Can you work these out from the model? Positions are in its coordinate system, mm. Face numbers are marked on the shaded views. A direction names the side the tool comes from. Give positions to 0.01 mm unless a question says otherwise; leave off trailing zeros. Loops run counter-clockwise (first coordinate to the right, second up) from the corner with the lowest first, then second, coordinate; pieces in that order, holes last. Notation, with made-up numbers: (29, -20) - (84, -20) arc R33 ccw to (84, 16) - close; hole circle Ø7 at (76.25, 5). An arc over 180 degrees is marked (long way). Answer as a JSON object with one key per item and string values. Group by question number.
Item 1: Which directions (+Z, -Z, +X, -X, +Y, -Y) give clear straight access to the entire face, cutting with the end or side of a thin tool? Please do the marked faces 1, 2 and 3.
Item 2: Suppose I cut it at D-D on z = 83. Write out the boundary of the cut face in (x, y).
Item 3: Thinking about a two-plate mould opening in X: for the marked faces 4, 5 and 6, which applies, pulls with the +X half, pulls with the -X half, needs draft (parallel to the pull), parting line crosses it, or undercut?
Item 4: Please list where these lines run through material, in increasing order: L1, parallel to Z at x = -124, y = 75.5; L2, parallel to Y at x = -50, z = 27; L3, parallel to X at y = 6, z = 104.5.
Item 5: Suppose I cut it at A-A on x = -80. Write out the boundary of the cut face in (y, z), and give its area (3 significant figures).
Item 6: Suppose I cut it at C-C on x = -60. Write out the boundary of the cut face in (y, z), and give its area (4 significant figures).
Item 7: Will these pins go through, and if not, where does the flat tip stop? pin 1 (2 mm diameter, centred on y = 26.5, z = 50, fed in from -X); pin 2 (6 mm diameter, centred on x = -67.47, z = 27.53, fed in from +Y).
Item 8: Suppose I cut it at B-B on z = 97.53. Write out the boundary of the cut face in (x, y), and give its area (3 significant figures).
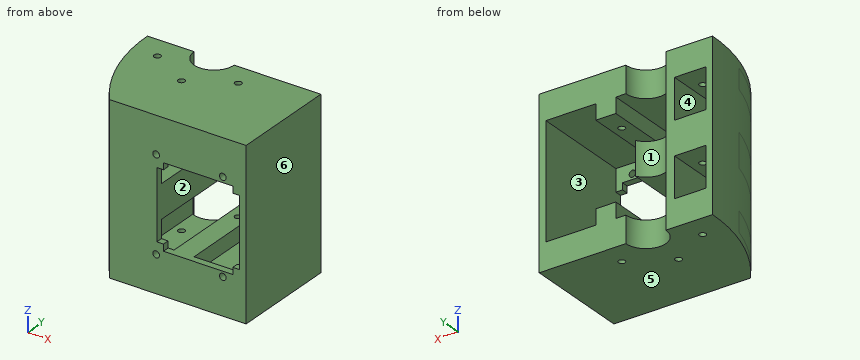
Autodesk Inventor part; units mm, degrees
ref_plane "YZ Plane" through (0, 0, 0) normal (1, 0, 0) x (0, 1, 0)
ref_plane "XZ Plane" through (0, 0, 0) normal (0, 1, 0) x (-1, 0, 0)
ref_plane "XY Plane" through (0, 0, 0) normal (0, 0, 1) x (1, 0, 0)
sketch "Sketch1" plane through (0, 0, 0) normal (0, 0, 1) x (1, 0, 0)
  circle A0 centre (0, 80) radius 130 construction
  line L0 (0, -50) -> (0, 0) construction
  line L1 (0, 0) -> (-102.4695, 0) construction
  arc A1 (-130, 80) -> (-102.4695, 0) centre (0, 80) ccw
  line L2 (-130, 80) -> (0, 80)
  line L3 (0, 80) -> (0, 0)
  line L4 (-102.4695, 0) -> (0, 0)
  dimension "d0" = 260
  dimension "d1" = 50
extrude "Extrusion1" add sketch "Sketch1" along normal blind 125
sketch "Sketch6" plane through (-130, 80, 0) normal (0, 1, 0) x (1, 0, 0)
  line L0 (0, 0) -> (0, -125)
  line L1 (0, 0) -> (130, 0)
  line L2 (130, 0) -> (130, -125)
  line L3 (130, -125) -> (0, -125)
  line L4 (0, -125) -> (0, 0)
  line L5 (5, -120) -> (125, -120)
  line L6 (125, -120) -> (125, -5)
  line L7 (125, -5) -> (5, -5)
  line L8 (5, -5) -> (5, -120)
  point P0 (130, 0)
  dimension "d25" = 5
extrude "Extrusion5" cut sketch "Sketch6" against normal blind 75 contours L8 L7 L6 L5
sketch "Sketch7" plane through (-102.4695, 0, 0) normal (0, -1, 0) x (1, 0, 0)
  circle A0 centre (35, 97.53) radius 2.5
  circle A1 centre (85, 97.53) radius 2.5
  line L0 (0, 125) -> (102.4695, 125)
  line L1 (0, 0) -> (0, 125)
  circle A2 centre (35, 27.53) radius 2.5
  circle A3 centre (85, 27.53) radius 2.5
  line L2 (102.4695, 0) -> (102.4695, 125)
  dimension "d28" = 5
  dimension "d29" = 5
  dimension "d30" = 27.47
  dimension "d31" = 50
  dimension "d33" = 5
  dimension "d34" = 5
  dimension "d35" = 70
  dimension "d82" = 35
extrude "Extrusion6" cut sketch "Sketch7" against normal through all
sketch "Sketch8" plane through (0, 0, 125) normal (0, 0, 1) x (1, 0, 0)
  line L0 (0, 80) -> (-130, 80)
  arc A0 (-130, 80) -> (-102.4695, 0) centre (0, 80) ccw
  arc A1 (-130, 80) -> (-102.4695, 0) centre (9.9581, 83.4269) ccw
  line L1 (-102.4695, 0) -> (-97.4695, 0)
  line L2 (-102.4695, 0) -> (0, 0)
  line L3 (-130, 80) -> (-125, 80)
  arc A2 (-125, 80) -> (-97.4695, 0) centre (14.9581, 83.4269) ccw
  dimension "d40" = 5
  dimension "d41" = 5
  dimension "d42" = 140
extrude "Extrusion7" add sketch "Sketch8" against normal blind 125
sketch "Sketch11" plane through (-130, 5, 0) normal (0, 1, 0) x (1, 0, 0)
  line L0 (125, -5) -> (125, -120)
  line L1 (125, -50) -> (5, -50)
  line L2 (5, -50) -> (5, -65)
  line L3 (5, -65) -> (125, -65)
  line L4 (125, -65) -> (125, -50)
  line L5 (125, -60) -> (5, -60)
  line L6 (5, -60) -> (5, -75)
  line L7 (5, -75) -> (125, -75)
  line L8 (125, -75) -> (125, -60)
  line L9 (32.7619, 0) -> (32.7619, -150)
  line L10 (125, -105) -> (5, -105)
  line L11 (5, -105) -> (5, -120)
  line L12 (5, -120) -> (125, -120)
  line L13 (125, -120) -> (125, -105)
  line L14 (125, -20) -> (5, -20)
  line L15 (5, -20) -> (5, -5)
  line L16 (5, -5) -> (125, -5)
  line L17 (125, -5) -> (125, -20)
  line L18 (5, -5) -> (125, -5)
  line L19 (5, -120) -> (5, -5)
  line L20 (125, -120) -> (5, -120)
  line L21 (125, -5) -> (125, -20)
  point P0 (130, 0)
  point P1 (65, -120)
  point P2 (65, -5)
  point P3 (5, -12.5)
  point P4 (5, -57.5)
  dimension "d54" = 15
  dimension "d55" = 15
  dimension "d56" = 15
  dimension "d57" = 15
  dimension "d58" = 30
  dimension "d59" = 30
  dimension "d66" = 5
extrude "Extrusion10" add sketch "Sketch11" along normal blind 75 contours L0 L14 L9 L16 | L9 L14 L15 L16 | L0 L5 L9 L1 | L0 L3 L9 L5 | L9 L5 L2 L1 | L0 L7 L9 L3 | L9 L3 L2 L5 | L9 L7 L6 L3 | L0 L12 L9 L10 | L9 L12 L11 L10
sketch "Sketch12" plane through (-130, 5, 0) normal (0, 1, 0) x (1, 0, 0)
  line L0 (27.5305, 0) -> (130, 0)
  line L1 (27.5305, -125) -> (130, -125)
  line L2 (72.5, 0) -> (87.5, 0)
  line L3 (87.5, 0) -> (87.5, -125)
  line L4 (87.5, -125) -> (72.5, -125)
  line L5 (72.5, -125) -> (72.5, 0)
  line L6 (28.5256, 0) -> (43.5256, 0)
  line L7 (43.5256, 0) -> (43.5256, -125)
  line L8 (43.5256, -125) -> (28.5256, -125)
  line L9 (28.5256, -125) -> (28.5256, 0)
  line L10 (130, 0) -> (130, -125)
  dimension "d62" = 15
  dimension "d63" = 15
  dimension "d92" = 42.5
extrude "Extrusion11" add sketch "Sketch12" along normal blind 75 contours L0 L7 L1 L9 | L0 L3 L1 L5
sketch "Sketch9" plane through (0, 0, 125) normal (0, 0, 1) x (1, 0, 0)
  circle A0 centre (-80, 80) radius 15
  point P0 (0, 0)
  point P1 (0, 80)
  dimension "d45" = 30
  dimension "d46" = 80
extrude "Extrusion8" cut sketch "Sketch9" against normal through all
sketch "Sketch13" plane through (0, 0, 0) normal (0, 0, -1) x (-1, 0, 0)
  arc A0 (102.4695, 0) -> (130, 80) centre (-9.9581, 83.4269) ccw
  line L0 (130, 80) -> (130, 80)
  arc A1 (102.4695, 0) -> (130, 80) centre (0, 80) ccw
  line L1 (130, 80) -> (130, 80)
  line L2 (95, 80) -> (130, 80)
  line L3 (130, 80) -> (130, 0)
  line L4 (130, 0) -> (102.4695, 0)
  point P0 (0, 0)
  dimension "d67" = 140
extrude "Extrusion12" cut sketch "Sketch13" against normal through all contours A1 L3 L4
sketch "Sketch14" plane through (0, 0, 125) normal (0, 0, 1) x (1, 0, 0)
  line L0 (-102.4695, 0) -> (0, 0) construction
  circle A0 centre (-110.3109, 97.5) radius 2.5
  circle A1 centre (-80, 80) radius 35 construction
  circle A2 centre (-110.3109, 62.5) radius 2.5
  circle A3 centre (-80, 45) radius 2.5
  circle A4 centre (-49.6891, 62.5) radius 2.5
  circle A5 centre (-49.6891, 97.5) radius 2.5
  circle A6 centre (-80, 115) radius 2.5
  arc A7 (-95, 80) -> (-65, 80) centre (-80, 80) ccw
  point P0 (0, 80)
  dimension "d74" = 70
  dimension "d72" = 5
  dimension "d77" = 360
extrude "Extrusion13" cut sketch "Sketch14" against normal through all
sketch "Sketch16" plane through (-102.4695, 0, 0) normal (0, -1, 0) x (1, 0, 0)
  line L0 (35.4695, 31.5) -> (35.4695, 93.5) construction
  line L1 (97.4695, 93.5) -> (35.4695, 93.5) construction
  line L2 (35.4695, 93.5) -> (35.4695, 31.5) construction
  line L3 (35.4695, 31.5) -> (97.4695, 31.5) construction
  line L4 (97.4695, 31.5) -> (97.4695, 93.5) construction
  line L5 (0, 125) -> (102.4695, 125)
  line L6 (0, 0) -> (102.4695, 0)
  line L7 (102.4695, 0) -> (102.4695, 125)
  line L8 (97.4695, 93.5) -> (92.4695, 93.5) construction
  line L9 (92.4695, 93.5) -> (92.4695, 88.5) construction
  line L10 (92.4695, 88.5) -> (97.4695, 88.5) construction
  line L11 (97.4695, 88.5) -> (97.4695, 93.5) construction
  line L12 (35.4695, 31.5) -> (40.4695, 31.5) construction
  line L13 (40.4695, 31.5) -> (40.4695, 36.5) construction
  line L14 (40.4695, 36.5) -> (35.4695, 36.5) construction
  line L15 (35.4695, 36.5) -> (35.4695, 31.5) construction
  line L16 (35.4695, 93.5) -> (40.4695, 93.5) construction
  line L17 (40.4695, 93.5) -> (40.4695, 88.5) construction
  line L18 (40.4695, 88.5) -> (35.4695, 88.5) construction
  line L19 (35.4695, 88.5) -> (35.4695, 93.5) construction
  line L20 (97.4695, 31.5) -> (92.4695, 31.5) construction
  line L21 (92.4695, 31.5) -> (92.4695, 36.5) construction
  line L22 (92.4695, 36.5) -> (97.4695, 36.5) construction
  line L23 (97.4695, 36.5) -> (97.4695, 31.5) construction
  line L24 (92.4695, 93.5) -> (40.4695, 93.5)
  line L25 (40.4695, 88.5) -> (40.4695, 93.5)
  line L26 (35.4695, 88.5) -> (40.4695, 88.5)
  line L27 (35.4695, 88.5) -> (35.4695, 36.5)
  line L28 (35.4695, 36.5) -> (40.4695, 36.5)
  line L29 (40.4695, 36.5) -> (40.4695, 31.5)
  line L30 (40.4695, 31.5) -> (92.4695, 31.5)
  line L31 (92.4695, 31.5) -> (92.4695, 36.5)
  line L32 (92.4695, 36.5) -> (97.4695, 36.5)
  line L33 (97.4695, 20) -> (97.4695, 50)
  line L34 (97.4695, 36.5) -> (97.4695, 88.5)
  line L35 (97.4695, 75) -> (97.4695, 105)
  line L36 (92.4695, 88.5) -> (97.4695, 88.5)
  line L37 (92.4695, 88.5) -> (92.4695, 93.5)
  point P0 (97.4695, 62.5)
  point P1 (102.4695, 62.5)
  point P2 (66.4695, 31.5)
  point P3 (51.2348, 0)
  dimension "d100" = 62
  dimension "d101" = 62
  dimension "d102" = 5
  dimension "d103" = 5
  dimension "d104" = 5
  dimension "d105" = 5
  dimension "d106" = 5
  dimension "d107" = 5
  dimension "d108" = 5
  dimension "d109" = 5
  dimension "d110" = 5
extrude "Extrusion15" cut sketch "Sketch16" against normal through all
equation "\"d101\" = d100"
properties part number "SJ005" material "ABS Plastic"
Worked out:
{
 "1": {"face 1": "+Z, -Z, +Y", "face 2": "+Y, -Y", "face 3": "+Y"},
 "2": {"outline": "(-130, 80) arc R130 ccw to (-102.47, 0) - (-67, 0) - (-67, 5) - (-86.47, 5) - (-86.47, 66.47) arc R15 cw to (-95, 80) - (-101.47, 80) - (-101.47, 5.69) arc R140 cw to (-125, 80) - close; (-5, 0) - (0, 0) - (0, 80) - (-5, 80) - close"},
 "3": {"face 4": "undercut", "face 5": "needs draft", "face 6": "pulls with the +X half"},
 "4": {"L1": "z = 0 to 20, 50 to 75, 105 to 125", "L2": "y = 0 to 60.02, 64.98 to 80", "L3": "x = -106.88 to -101.68, -101.47 to -86.47, -57.5 to -42.5, -5 to 0"},
 "5": {"outline": "(0, 0) - (42.5, 0) - (42.5, 20) - (5, 20) - (5, 50) - (42.5, 50) - (42.5, 75) - (5, 75) - (5, 105) - (42.5, 105) - (42.5, 125) - (0, 125) - close; (47.5, 0) - (65, 0) - (65, 20) - (47.5, 20) - close; (47.5, 50) - (65, 50) - (65, 75) - (47.5, 75) - close; (47.5, 105) - (65, 105) - (65, 125) - (47.5, 125) - close", "area": "4,200 mm2"},
 "6": {"outline": "(0, 0) - (80, 0) - (80, 20) - (5, 20) - (5, 31.5) - (0, 31.5) - close; (0, 93.5) - (5, 93.5) - (5, 105) - (80, 105) - (80, 125) - (0, 125) - close", "area": "3,315 mm2"},
 "7": {"pin 1": "stops at x = -118.93", "pin 2": "stops at y = 5"},
 "8": {"outline": "(-130, 80) arc R130 ccw to (-102.47, 0) - (-69.97, 0) - (-69.97, 5) - (-86.47, 5) - (-86.47, 66.47) arc R15 cw to (-95, 80) - (-101.47, 80) - (-101.47, 5.69) arc R140 cw to (-125, 80) - close; (-64.97, 0) - (-19.97, 0) - (-19.97, 5) - (-42.5, 5) - (-42.5, 80) - (-57.5, 80) - (-57.5, 5) - (-64.97, 5) - close; (-14.97, 0) - (0, 0) - (0, 80) - (-5, 80) - (-5, 5) - (-14.97, 5) - close; hole circle Ø5 at (-49.69, 62.5)", "area": "3,400 mm2"}
}
